Autodesk Inventor part; units mm, degrees
ref_plane "YZ Plane" through (0, 0, 0) normal (1, 0, 0) x (0, 1, 0)
ref_plane "XZ Plane" through (0, 0, 0) normal (0, 1, 0) x (-1, 0, 0)
ref_plane "XY Plane" through (0, 0, 0) normal (0, 0, 1) x (1, 0, 0)
sketch "Sketch1" plane through (0, 0, 0) normal (0, 1, 0) x (-1, 0, 0)
  line L0 (300, 300) -> (-300, 300)
  line L1 (-300, 300) -> (-300, -300)
  line L2 (-300, -300) -> (300, -300)
  line L3 (300, -300) -> (300, 300)
  line L4 (300, 300) -> (-300, -300) construction
  line L5 (-300, 300) -> (300, -300) construction
  line L6 (274.6, 274.6) -> (-274.6, 274.6)
  line L7 (-274.6, 274.6) -> (-274.6, -274.6)
  line L8 (-274.6, -274.6) -> (274.6, -274.6)
  line L9 (274.6, -274.6) -> (274.6, 274.6)
  line L10 (-70.84, -274.6) -> (-70.84, 274.6)
  line L11 (-96.24, 274.6) -> (-96.24, -274.6)
  line L12 (96.24, -274.6) -> (96.24, 274.6)
  line L13 (70.84, 274.6) -> (70.84, -274.6)
  line L14 (0, 0) -> (0, -274.6) construction
  dimension "d0" = 600
  dimension "d1" = 600
  dimension "d2" = 25.4
  dimension "d3" = 25.4
  dimension "d4" = 396.24
extrude "Extrusion1" add sketch "Sketch1" along normal blind 25.4 contours L3 L2 L1 L0 | L12 L8 L13 L6 | L10 L8 L11 L6
properties part number "MockChassis(delete asap)"
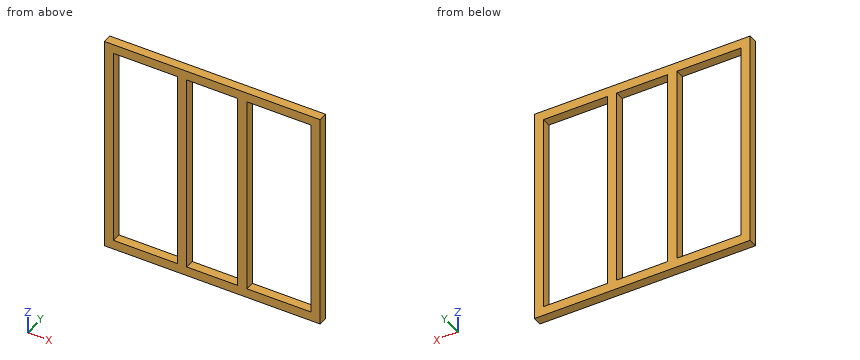
Part model, mm, in its own coordinate system. Coordinates: 2 decimals unless noted, no trailing zeros. Loops run counter-clockwise (first coordinate to the right, second up) from the corner with the lowest first, then second, coordinate; pieces in that order, holes last. Notation, with made-up numbers: (35, -18.75) - (58, -18.75) arc R20 cw to (58, 13.25) - close; hole circle Ø10 at (4.25, -6). An arc over 180 degrees is marked (long way). Write each question's results on one line, items separated by ' | '. Start each with the question number.
Q1. Slice it at B-B on y = 11.25. Give the cut face in (x, z), and give its area (3 significant figures).
Q2. Probe line 1 along X through (y, z) = (2.75, 10.5); line 2 along Z through (x, y) = (-201.5, 20). List the from-to ranges inside material, lowest first.
Q3. Slice it at A-A on x = -3.5. Give the cut face in (y, z), and give its area (3 significant figures).
Q4. Slice it at C-C on z = -101. Give the cut face in (x, y), and give its area (3 significant figures).
Answer:
1) outline: (-300, -300) - (300, -300) - (300, 300) - (-300, 300) - close; hole (-274.6, -274.6) - (-96.24, -274.6) - (-96.24, 274.6) - (-274.6, 274.6) - close; hole (-70.84, -274.6) - (70.84, -274.6) - (70.84, 274.6) - (-70.84, 274.6) - close; hole (96.24, -274.6) - (274.6, -274.6) - (274.6, 274.6) - (96.24, 274.6) - close | area: 86,300 mm2
2) line 1: x = -300 to -274.6, -96.24 to -70.84, 70.84 to 96.24, 274.6 to 300 | line 2: z = -300 to -274.6, 274.6 to 300
3) outline: (0, -300) - (25.4, -300) - (25.4, -274.6) - (0, -274.6) - close; (0, 274.6) - (25.4, 274.6) - (25.4, 300) - (0, 300) - close | area: 1,290 mm2
4) outline: (-300, 0) - (-274.6, 0) - (-274.6, 25.4) - (-300, 25.4) - close; (-96.24, 0) - (-70.84, 0) - (-70.84, 25.4) - (-96.24, 25.4) - close; (70.84, 0) - (96.24, 0) - (96.24, 25.4) - (70.84, 25.4) - close; (274.6, 0) - (300, 0) - (300, 25.4) - (274.6, 25.4) - close | area: 2,580 mm2
